Read the model definition and answer for the solid it produces. Units are mm, in the model's axes. A direction names the side the tool comes from. Give positions to 0.01 mm unless a question says otherwise; leave off trailing zeros. Write each loop counter-clockwise with the first axis right and the second up, starting at its lowest first coordinate (ties: lowest second). Pieces come first, ordered by that corner, then holes. Notation, with made-up numbers: (65.25, 23) -> (105.25, 23) arc R20 cw to (105.25, 35) -> close; hole circle Ø9 at (-19.75, 83). An arc over 180 degrees is marked (long way). Use a Markdown table: item, result.
from build123d import *

# Parameters (mm, degrees)
SKETCH1_R                            = 95.25
SKETCH1_R_2                          = 88.9
BOSS_EXTRUDE1_DEPTH                  = 50.8
SKETCH4_R                            = 3.175
CUT_EXTRUDE2_DEPTH                   = 10.16
BOSS_EXTRUDE3_DEPTH                  = 10.16
BOSS_EXTRUDE3_DIRECTION_2_REACH      = 220.96
BOSS_EXTRUDE3_DIRECTION_2_END_RADIUS = 95.25
BOSS_EXTRUDE9_REACH                  = 220.96
BOSS_EXTRUDE9_END_RADIUS             = 95.25
BOSS_EXTRUDE9_DIRECTION_2_DEPTH      = 0.254
SKETCH7_R                            = 3.175
CUT_EXTRUDE3_DEPTH                   = 220.180955111
BOSS_EXTRUDE10_START                 = -0.850464
SKETCH8_R                            = 12.7
SKETCH8_R_2                          = 3.175
BOSS_EXTRUDE10_DEPTH                 = 19.900464


with BuildPart() as part:
    # Sketch1 → Boss-Extrude1 (new body)
    with BuildSketch(Plane(origin=(0, 0, 0), x_dir=(1, 0, 0), z_dir=(0, 1, 0))):
        with Locations(Location((0, 0, 0), (0, 0, 270))):
            Circle(SKETCH1_R)
        with Locations(Location((0, 0, 0), (0, 0, 270))):
            Circle(SKETCH1_R_2, mode=Mode.SUBTRACT)
    extrude(amount=BOSS_EXTRUDE1_DEPTH)

    # Sketch4 → Cut-Extrude2 (cut)
    with BuildSketch(Plane(origin=(0, 0, -95.25), x_dir=(-1, 0, 0), z_dir=(0, 0, -1))):
        with Locations(Location((0, 25.4, 0), (0, 0, 90))):
            Circle(SKETCH4_R)
    cut_extrude2 = extrude(amount=-CUT_EXTRUDE2_DEPTH, mode=Mode.SUBTRACT)

    # Mirror2: Cut-Extrude2 across plane
    add(cut_extrude2.mirror(Plane.XY), mode=Mode.SUBTRACT)

    # Sketch5 → Boss-Extrude3 (add)
    with BuildSketch(Plane(origin=(95.25, 0, 0), x_dir=(0, 0, -1), z_dir=(1, 0, 0))):
        Polygon((14.732, 11.14102204), (10.902119397, 8.255), (10.902119397, 3.175), (-10.902119397, 3.175), (-10.902119397, 8.255), (-14.732, 11.14102204), (-17.272, 11.14102204), (-17.272, 9.874624755), (-13.442119397, 6.988602716), (-13.442119397, 0.635), (13.442119397, 0.635), (13.442119397, 6.988602716), (17.272, 9.874624755), (17.272, 11.14102204), align=None)
        with BuildLine():
            Line((17.272, 31.524764922), (17.272, 31.20702204))
            Line((17.272, 31.20702204), (14.732, 31.20702204))
            ThreePointArc((14.732, 31.20702204), (0, 42.545), (-14.732, 31.20702204))
            Line((-14.732, 31.20702204), (-17.272, 31.20702204))
            Line((-17.272, 31.20702204), (-17.272, 31.524764922))
            ThreePointArc((-17.272, 31.524764922), (0, 45.085), (17.272, 31.524764922))
        make_face()
    extrude(amount=BOSS_EXTRUDE3_DEPTH)

    # Boss-Extrude3 direction 2: up to this cylinder (the profile starts outside it)
    boss_extrude3_direction_2_end = Plane(origin=(0, 20.387773, 0), z_dir=(0, -1, 0)) * Cylinder(BOSS_EXTRUDE3_DIRECTION_2_END_RADIUS, 655.37624, mode=Mode.PRIVATE)
    # Sketch5 → Boss-Extrude3 direction 2 (add, up to the surface)
    with BuildSketch(Plane(origin=(95.25, 0, 0), x_dir=(0, 0, -1), z_dir=(1, 0, 0)), mode=Mode.PRIVATE) as boss_extrude3_direction_2_sk1:
        Polygon((14.732, 11.14102204), (10.902119397, 8.255), (10.902119397, 3.175), (-10.902119397, 3.175), (-10.902119397, 8.255), (-14.732, 11.14102204), (-17.272, 11.14102204), (-17.272, 9.874624755), (-13.442119397, 6.988602716), (-13.442119397, 0.635), (13.442119397, 0.635), (13.442119397, 6.988602716), (17.272, 9.874624755), (17.272, 11.14102204), align=None)
    boss_extrude3_direction_2_tool1 = extrude(boss_extrude3_direction_2_sk1.sketch, amount=-BOSS_EXTRUDE3_DIRECTION_2_REACH, mode=Mode.PRIVATE) - boss_extrude3_direction_2_end
    add(boss_extrude3_direction_2_tool1.solids().sort_by_distance((95.25, 9.409653, -13.034353))[0])
    add(boss_extrude3_direction_2_tool1.solids().sort_by_distance((95.25, 9.409653, -13.034353))[1])
    # Sketch5 → Boss-Extrude3 direction 2 (add, up to the surface)
    with BuildSketch(Plane(origin=(95.25, 0, 0), x_dir=(0, 0, -1), z_dir=(1, 0, 0)), mode=Mode.PRIVATE) as boss_extrude3_direction_2_sk2:
        with BuildLine():
            Line((17.272, 31.524764922), (17.272, 31.20702204))
            Line((17.272, 31.20702204), (14.732, 31.20702204))
            ThreePointArc((14.732, 31.20702204), (0, 42.545), (-14.732, 31.20702204))
            Line((-14.732, 31.20702204), (-17.272, 31.20702204))
            Line((-17.272, 31.20702204), (-17.272, 31.524764922))
            ThreePointArc((-17.272, 31.524764922), (0, 45.085), (17.272, 31.524764922))
        make_face()
    boss_extrude3_direction_2_tool2 = extrude(boss_extrude3_direction_2_sk2.sketch, amount=-BOSS_EXTRUDE3_DIRECTION_2_REACH, mode=Mode.PRIVATE) - boss_extrude3_direction_2_end
    add(boss_extrude3_direction_2_tool2.solids().sort_by_distance((95.25, 31.365893, -16.899725))[0])
    add(boss_extrude3_direction_2_tool2.solids().sort_by_distance((95.25, 31.365893, -16.899725))[1])

    # Boss-Extrude9: up to this cylinder (the profile starts outside it)
    boss_extrude9_end = Plane(origin=(0, 22.775292, 0), z_dir=(0, -1, 0)) * Cylinder(BOSS_EXTRUDE9_END_RADIUS, 633.42, mode=Mode.PRIVATE)
    # Sketch6 → Boss-Extrude9 (add, up to the surface)
    with BuildSketch(Plane(origin=(95.25, 0, 0), x_dir=(0, 0, -1), z_dir=(1, 0, 0)), mode=Mode.PRIVATE) as boss_extrude9_sk1:
        with BuildLine():
            Line((15.720104226, 32.350634064), (24.376259803, 31.134090734))
            ThreePointArc((24.376259803, 31.134090734), (29.020776957, 26.241656743), (25.300667362, 20.614203096))
            Line((25.300667362, 20.614203096), (16.002, 17.585051702))
            Line((16.002, 17.585051702), (16.002, 10.507823398))
            Line((16.002, 10.507823398), (12.172119397, 7.621801358))
            Line((12.172119397, 7.621801358), (12.172119397, 1.905))
            Line((12.172119397, 1.905), (-12.172119397, 1.905))
            Line((-12.172119397, 1.905), (-12.172119397, 7.621801358))
            Line((-12.172119397, 7.621801358), (-16.002, 10.507823398))
            Line((-16.002, 10.507823398), (-16.002, 17.585051702))
            Line((-16.002, 17.585051702), (-25.300667362, 20.614203096))
            ThreePointArc((-25.300667362, 20.614203096), (-29.020776957, 26.241656743), (-24.376259803, 31.134090734))
            Line((-24.376259803, 31.134090734), (-15.720104226, 32.350634064))
            ThreePointArc((-15.720104226, 32.350634064), (0, 43.815), (15.720104226, 32.350634064))
        make_face()
    boss_extrude9_tool1 = extrude(boss_extrude9_sk1.sketch, amount=-BOSS_EXTRUDE9_REACH, mode=Mode.PRIVATE) - boss_extrude9_end
    add(boss_extrude9_tool1.solids().sort_by_distance((95.25, 22.775292, 0))[0])
    add(boss_extrude9_tool1.solids().sort_by_distance((95.25, 22.775292, 0))[1])

    # Sketch6 → Boss-Extrude9 direction 2 (add)
    with BuildSketch(Plane(origin=(95.25, 0, 0), x_dir=(0, 0, -1), z_dir=(1, 0, 0))):
        with BuildLine():
            Line((15.720104226, 32.350634064), (24.376259803, 31.134090734))
            ThreePointArc((24.376259803, 31.134090734), (29.020776957, 26.241656743), (25.300667362, 20.614203096))
            Line((25.300667362, 20.614203096), (16.002, 17.585051702))
            Line((16.002, 17.585051702), (16.002, 10.507823398))
            Line((16.002, 10.507823398), (12.172119397, 7.621801358))
            Line((12.172119397, 7.621801358), (12.172119397, 1.905))
            Line((12.172119397, 1.905), (-12.172119397, 1.905))
            Line((-12.172119397, 1.905), (-12.172119397, 7.621801358))
            Line((-12.172119397, 7.621801358), (-16.002, 10.507823398))
            Line((-16.002, 10.507823398), (-16.002, 17.585051702))
            Line((-16.002, 17.585051702), (-25.300667362, 20.614203096))
            ThreePointArc((-25.300667362, 20.614203096), (-29.020776957, 26.241656743), (-24.376259803, 31.134090734))
            Line((-24.376259803, 31.134090734), (-15.720104226, 32.350634064))
            ThreePointArc((-15.720104226, 32.350634064), (0, 43.815), (15.720104226, 32.350634064))
        make_face()
    extrude(amount=BOSS_EXTRUDE9_DIRECTION_2_DEPTH)

    # Sketch7 → Cut-Extrude3 (cut, through all)
    with BuildSketch(Plane(origin=(95.504, 0, 0), x_dir=(0, 0, -1), z_dir=(1, 0, 0))):
        with Locations((0, 25.4)):
            Circle(SKETCH7_R)
    extrude(amount=-CUT_EXTRUDE3_DEPTH, mode=Mode.SUBTRACT)

    # Sketch8 → Boss-Extrude10 (add)
    with BuildSketch(Plane(origin=(0, 0, -95.25), x_dir=(-1, 0, 0), z_dir=(0, 0, -1)).offset(BOSS_EXTRUDE10_START)):
        with Locations(Location((0, 25.4, 0), (0, 0, 90))):
            Circle(SKETCH8_R)
        with Locations((0, 25.4)):
            Circle(SKETCH8_R_2, mode=Mode.SUBTRACT)
    boss_extrude10 = extrude(amount=BOSS_EXTRUDE10_DEPTH)

    # Mirror3: Boss-Extrude10 across plane
    add(boss_extrude10.mirror(Plane.XY))


solid = part.part
Item 1: A cutting plane is placed at D-D (x = -30). Give the vertices of the cut face in (y, z), then the cut area to 3 significant figures.
Return value:
| item | result |
|---|---|
| outline | (0, -90.4) -> (50.8, -90.4) -> (50.8, -83.69) -> (0, -83.69) -> close; (0, 83.69) -> (50.8, 83.69) -> (50.8, 90.4) -> (0, 90.4) -> close |
| area | 682 mm^2 |
Item 2: A cutting plane is placed at A-A (x = 0). Give the vertices of the cut face in (y, z) (3 decimals).
Return value:
| item | result |
|---|---|
| outline | (0, -95.25) -> (12.7, -95.25) -> (12.7, -114.3) -> (22.225, -114.3) -> (22.225, -88.9) -> (0, -88.9) -> close; (0, 88.9) -> (22.225, 88.9) -> (22.225, 114.3) -> (12.7, 114.3) -> (12.7, 95.25) -> (0, 95.25) -> close; (28.575, -114.3) -> (38.1, -114.3) -> (38.1, -95.25) -> (50.8, -95.25) -> (50.8, -88.9) -> (28.575, -88.9) -> close; (28.575, 88.9) -> (50.8, 88.9) -> (50.8, 95.25) -> (38.1, 95.25) -> (38.1, 114.3) -> (28.575, 114.3) -> close |
Item 3: Straight lines are drawn through the part: line 1 along Z through (x, y) = (-2, 41); line 2 along Y through (x, z) = (91, 0) (3 decimals); line 3 along X through (y, z) = (25, -99). For each, find the intervals that lie inside material, in ascending order. Write a range as [from, to].
Return value:
| item | result |
|---|---|
| line 1 | [-95.23, -88.88], [88.88, 95.23] |
| line 2 | [0, 22.225], [28.575, 50.8] |
| line 3 | [-12.69, -3.15], [3.15, 12.69] |
Item 4: For a pull along Y with two mould halves and no side action, classify faces 1 (the face through (92.22, 28.55, 0.41)), 2 (the face through (93.08, 26.14, 29.03)), 3 (the face through (105.41, 2, 0)), 4 (the face through (101, 3.175, 0)) as +Y half, -Y half, draft (parallel to the pull), parting line (faces both ways), or undercut.
Return value:
| item | result |
|---|---|
| face 1 | undercut |
| face 2 | parting line |
| face 3 | draft |
| face 4 | undercut |
Item 5: A tool of negligible diameter and unlimited length cuts with its end or side. For faces 5 (the face through (100, 4, 13.442)), 6 (the face through (93.08, 26.34, -29.01)), 7 (the face through (100, 4, -13.442)), from which of +Z, -Z, +X, -X, +Y, -Y can it reach the whole face along a straight path? Write none if from no direction.
Return value:
| item | result |
|---|---|
| face 5 | +Z, +X, -Y |
| face 6 | -Z, +X |
| face 7 | -Z, +X, -Y |
Item 6: Each of these flat-tipped pins is pushed along its axis until it touches: P1, Ø6, axis at x = -56.5, y = 37, coming from the +Z side; P2, Ø5.5, axis at x = 98.5, z = -3, coming from the -Y side (3 decimals); P3, Ø6, axis at y = 31, z = 87.5, coming from the +X side. Where does it stop, or does it pass through?
Return value:
| item | result |
|---|---|
| P1 | z = 78.81 |
| P2 | y = 0.635 |
| P3 | x = 43.96 |
Item 7: A cutting plane is placed at C-C (z = 77.5). Give the vertices of the cut face in (x, y).
Return value:
| item | result |
|---|---|
| outline | (-55.37, 0) -> (-43.55, 0) -> (-43.55, 50.8) -> (-55.37, 50.8) -> close; (43.55, 0) -> (55.37, 0) -> (55.37, 50.8) -> (43.55, 50.8) -> close |
Item 8: A cutting plane is placed at B-B (y = 25.4). Give the vertices of the cut face in (x, z) (3 decimals), then the cut area to 3 significant figures.
Return value:
| item | result |
|---|---|
| outline | (-95.197, -3.175) arc R95.25 ccw to (-12.7, -94.4) -> (-12.7, -114.3) -> (-3.175, -114.3) -> (-3.175, -88.843) arc R88.9 cw to (-88.843, -3.175) -> close; (-95.197, 3.175) -> (-88.843, 3.175) arc R88.9 cw to (-3.175, 88.843) -> (-3.175, 114.3) -> (-12.7, 114.3) -> (-12.7, 94.4) arc R95.25 ccw to start; (3.175, -114.3) -> (12.7, -114.3) -> (12.7, -94.4) arc R95.25 ccw to (90.719, -29.029) -> (95.504, -29.029) -> (95.504, -3.175) -> (88.843, -3.175) arc R88.9 cw to (3.175, -88.843) -> close; (3.175, 88.843) arc R88.9 cw to (88.843, 3.175) -> (95.504, 3.175) -> (95.504, 29.029) -> (90.719, 29.029) arc R95.25 ccw to (12.7, 94.4) -> (12.7, 114.3) -> (3.175, 114.3) -> close |
| area | 4,350 mm^2 |
